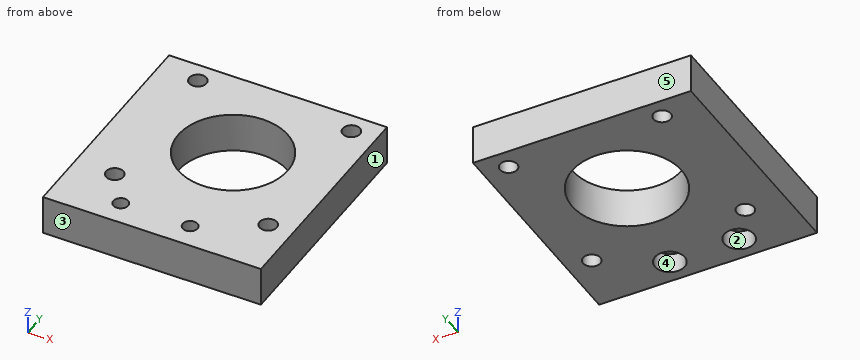
from build123d import *

# Parameters (mm, degrees)
SKETCH_1_W          = 8
SKETCH_1_H          = 47
EXTRUDE_1_DEPTH     = 44
CUT_EXTRUDE_1_REACH = 61.141
SKETCH_2_R          = 11.05
SKETCH_2_R_2        = 1.75
SKETCH_2_R_3        = 1.5
SKETCH_6_R          = 3
CUT_EXTRUDE_3_DEPTH = 4


with BuildPart() as part:
    # 草图1 → 凸台-拉伸1 (new body)
    with BuildSketch(Plane(origin=(0, 0, 0), x_dir=(0, 0, -1), z_dir=(1, 0, 0))):
        with Locations((-0.573456279, 15.2)):
            Rectangle(SKETCH_1_W, SKETCH_1_H)
    extrude(amount=-EXTRUDE_1_DEPTH)

    # 草图2 → 切除-拉伸1 (cut, up to next)
    with BuildSketch(Plane(origin=(0, 0, -3.426543721), x_dir=(-1, 0, 0), z_dir=(0, 0, -1)), mode=Mode.PRIVATE) as cut_extrude_1_sk1:
        with Locations(Location((20.5, 19.159060435, 0), (0, 0, 90))):
            Circle(SKETCH_2_R)
    cut_extrude_1_tool1 = extrude(cut_extrude_1_sk1.sketch, amount=-CUT_EXTRUDE_1_REACH, mode=Mode.PRIVATE) & part.part
    # 草图2 → 切除-拉伸1 (cut, up to next)
    with BuildSketch(Plane(origin=(0, 0, -3.426543721), x_dir=(-1, 0, 0), z_dir=(0, 0, -1)), mode=Mode.PRIVATE) as cut_extrude_1_sk2:
        with Locations(Location((5, 34.659060435, 0), (0, 0, 90))):
            Circle(SKETCH_2_R_2)
    cut_extrude_1_tool2 = extrude(cut_extrude_1_sk2.sketch, amount=-CUT_EXTRUDE_1_REACH, mode=Mode.PRIVATE) & part.part
    # 草图2 → 切除-拉伸1 (cut, up to next)
    with BuildSketch(Plane(origin=(0, 0, -3.426543721), x_dir=(-1, 0, 0), z_dir=(0, 0, -1)), mode=Mode.PRIVATE) as cut_extrude_1_sk3:
        with Locations(Location((5, 3.659060435, 0), (0, 0, 90))):
            Circle(SKETCH_2_R_2)
    cut_extrude_1_tool3 = extrude(cut_extrude_1_sk3.sketch, amount=-CUT_EXTRUDE_1_REACH, mode=Mode.PRIVATE) & part.part
    # 草图2 → 切除-拉伸1 (cut, up to next)
    with BuildSketch(Plane(origin=(0, 0, -3.426543721), x_dir=(-1, 0, 0), z_dir=(0, 0, -1)), mode=Mode.PRIVATE) as cut_extrude_1_sk4:
        with Locations(Location((36, 3.659060435, 0), (0, 0, 90))):
            Circle(SKETCH_2_R_2)
    cut_extrude_1_tool4 = extrude(cut_extrude_1_sk4.sketch, amount=-CUT_EXTRUDE_1_REACH, mode=Mode.PRIVATE) & part.part
    # 草图2 → 切除-拉伸1 (cut, up to next)
    with BuildSketch(Plane(origin=(0, 0, -3.426543721), x_dir=(-1, 0, 0), z_dir=(0, 0, -1)), mode=Mode.PRIVATE) as cut_extrude_1_sk5:
        with Locations(Location((36, 34.659060435, 0), (0, 0, 90))):
            Circle(SKETCH_2_R_2)
    cut_extrude_1_tool5 = extrude(cut_extrude_1_sk5.sketch, amount=-CUT_EXTRUDE_1_REACH, mode=Mode.PRIVATE) & part.part
    # 草图2 → 切除-拉伸1 (cut, up to next)
    with BuildSketch(Plane(origin=(0, 0, -3.426543721), x_dir=(-1, 0, 0), z_dir=(0, 0, -1)), mode=Mode.PRIVATE) as cut_extrude_1_sk6:
        with Locations(Location((17, -3.3, 0), (0, 0, 90))):
            Circle(SKETCH_2_R_3)
    cut_extrude_1_tool6 = extrude(cut_extrude_1_sk6.sketch, amount=-CUT_EXTRUDE_1_REACH, mode=Mode.PRIVATE) & part.part
    # 草图2 → 切除-拉伸1 (cut, up to next)
    with BuildSketch(Plane(origin=(0, 0, -3.426543721), x_dir=(-1, 0, 0), z_dir=(0, 0, -1)), mode=Mode.PRIVATE) as cut_extrude_1_sk7:
        with Locations(Location((31, -3.3, 0), (0, 0, 90))):
            Circle(SKETCH_2_R_3)
    cut_extrude_1_tool7 = extrude(cut_extrude_1_sk7.sketch, amount=-CUT_EXTRUDE_1_REACH, mode=Mode.PRIVATE) & part.part
    add(cut_extrude_1_tool1.solids().sort_by_distance((-20.5, 19.15906, -3.426544))[0], mode=Mode.SUBTRACT)
    add(cut_extrude_1_tool2.solids().sort_by_distance((-5, 34.65906, -3.426544))[0], mode=Mode.SUBTRACT)
    add(cut_extrude_1_tool3.solids().sort_by_distance((-5, 3.65906, -3.426544))[0], mode=Mode.SUBTRACT)
    add(cut_extrude_1_tool4.solids().sort_by_distance((-36, 3.65906, -3.426544))[0], mode=Mode.SUBTRACT)
    add(cut_extrude_1_tool5.solids().sort_by_distance((-36, 34.65906, -3.426544))[0], mode=Mode.SUBTRACT)
    add(cut_extrude_1_tool6.solids().sort_by_distance((-17, -3.3, -3.426544))[0], mode=Mode.SUBTRACT)
    add(cut_extrude_1_tool7.solids().sort_by_distance((-31, -3.3, -3.426544))[0], mode=Mode.SUBTRACT)

    # 草图6 → 切除-拉伸3 (cut)
    with BuildSketch(Plane(origin=(0, 0, -3.426543721), x_dir=(-1, 0, 0), z_dir=(0, 0, -1))):
        with Locations(Location((17, -3.3, 0), (0, 0, 90))):
            Circle(SKETCH_6_R)
        with Locations(Location((31, -3.3, 0), (0, 0, 90))):
            Circle(SKETCH_6_R)
    extrude(amount=-CUT_EXTRUDE_3_DEPTH, mode=Mode.SUBTRACT)


solid = part.part
Input: part model. Units: mm. Frame: model coordinates. Face numbers are marked on the shaded views. A direction names the side the tool comes from. Round coordinates to 2 decimals unless told otherwise and drop trailing zeros. Order: outer loops, then holes, each group sorted by start corner. A loop starts at its lowest first (then second) coordinate and runs counter-clockwise, first axis right, second up. Notation, with made-up numbers: (12.25, 55.5) - (29.25, 55.5) arc R7 ccw to (29.25, 67.5) - close; hole circle Ø11 at (-15.75, -29). An arc over 180 degrees is marked (long way). Use a Markdown table: item, result.
1. Section C-C on z = -0.25. Return the cut outline in (x, y).
Evaluation:
| item | result |
|---|---|
| outline | (-44, -8.3) - (0, -8.3) - (0, 38.7) - (-44, 38.7) - close; hole circle Ø3.5 at (-36, 3.66); hole circle Ø3.5 at (-36, 34.66); hole circle Ø6 at (-31, -3.3); hole circle Ø22.1 at (-20.5, 19.16); hole circle Ø6 at (-17, -3.3); hole circle Ø3.5 at (-5, 3.66); hole circle Ø3.5 at (-5, 34.66) |
2. Section A-A on y = -3.3. Return the cut outline in (x, z), then the cut area to 3 significant figures.
Evaluation:
| item | result |
|---|---|
| outline | (-44, -3.43) - (-34, -3.43) - (-34, 0.57) - (-32.5, 0.57) - (-32.5, 4.57) - (-44, 4.57) - close; (-29.5, 0.57) - (-28, 0.57) - (-28, -3.43) - (-20, -3.43) - (-20, 0.57) - (-18.5, 0.57) - (-18.5, 4.57) - (-29.5, 4.57) - close; (-15.5, 0.57) - (-14, 0.57) - (-14, -3.43) - (0, -3.43) - (0, 4.57) - (-15.5, 4.57) - close |
| area | 280 mm^2 |
3. Mould query, pull axis Y, two halves, no side actions, for the marked faces 1, 2 and 3. Classes: +Y half, -Y half, draft (parallel to the pull), parting line (faces both ways), or undercut.
Evaluation:
| item | result |
|---|---|
| face 1 | draft |
| face 2 | undercut |
| face 3 | -Y half |
4. First-contact query: pin 1 (5.5 mm diameter, centred on x = -31, y = -3.3, fed in from -Z). Flat tip, straight axial feed; report the tip coordinate or a pass-through.
Evaluation:
| item | result |
|---|---|
| pin 1 | z = 0.57 |
5. Section B-B on x = -36. Return the cut outline in (y, z).
Evaluation:
| item | result |
|---|---|
| outline | (-8.3, -3.43) - (1.91, -3.43) - (1.91, 4.57) - (-8.3, 4.57) - close; (5.41, -3.43) - (32.91, -3.43) - (32.91, 4.57) - (5.41, 4.57) - close; (36.41, -3.43) - (38.7, -3.43) - (38.7, 4.57) - (36.41, 4.57) - close |
6. Access query for the marked faces 4 and 5. Directions: +Z, -Z, +X, -X, +Y, -Y. A direction counts if a zero-diameter tool reaches every point of the face in a straight line with its end or side. Return the directions, or none.
Evaluation:
| item | result |
|---|---|
| face 4 | -Z |
| face 5 | +Z, -Z, +X, -X, +Y |
7. Material intervals for probe 1 along X at (y, z) = (-3.3, -2.6); probe 2 along Y at (x, z) = (-16, 2.75); probe 3 along Y at (x, z) = (-19, -1), sorted ascending.
Evaluation:
| item | result |
|---|---|
| probe 1 | -44 to -34, -28 to -20, -14 to 0 |
| probe 2 | -8.3 to -4.42, -2.18 to 9.07, 29.25 to 38.7 |
| probe 3 | -8.3 to -5.54, -1.06 to 8.21, 30.11 to 38.7 |
8. Section D-D on x = -10.5. Return the cut outline in (y, z).
Evaluation:
| item | result |
|---|---|
| outline | (-8.3, -3.43) - (14.46, -3.43) - (14.46, 4.57) - (-8.3, 4.57) - close; (23.86, -3.43) - (38.7, -3.43) - (38.7, 4.57) - (23.86, 4.57) - close |
